```python
from build123d import *

# Parameters (mm, degrees)
BOSS_EXTRUDE1_DEPTH = 2.5
SKETCH2_R           = 1.75
SKETCH2_W           = 3.5
SKETCH2_H           = 6.7
CUT_EXTRUDE1_DEPTH  = 2.5


with BuildPart() as part:
    # Sketch1 → Boss-Extrude1 (new body)
    with BuildSketch(Plane(origin=(0, 0, 0), x_dir=(1, 0, 0), z_dir=(0, 1, 0))):
        Polygon((5.3, 0), (-5.3, 0), (-5.3, 41.8), (-7.6, 41.8), (-7.6, 46.6), (7.6, 46.6), (7.6, 41.8), (5.3, 41.8), align=None)
    extrude(amount=BOSS_EXTRUDE1_DEPTH)

    # Sketch2 → Cut-Extrude1 (cut)
    with BuildSketch(Plane(origin=(0, 0, 0), x_dir=(1, 0, 0), z_dir=(0, 1, 0))):
        with Locations((0, 3.2)):
            Circle(SKETCH2_R)
        with Locations((0, 20.75)):
            Rectangle(SKETCH2_W, SKETCH2_H)
    extrude(amount=CUT_EXTRUDE1_DEPTH, mode=Mode.SUBTRACT)


solid = part.part
```
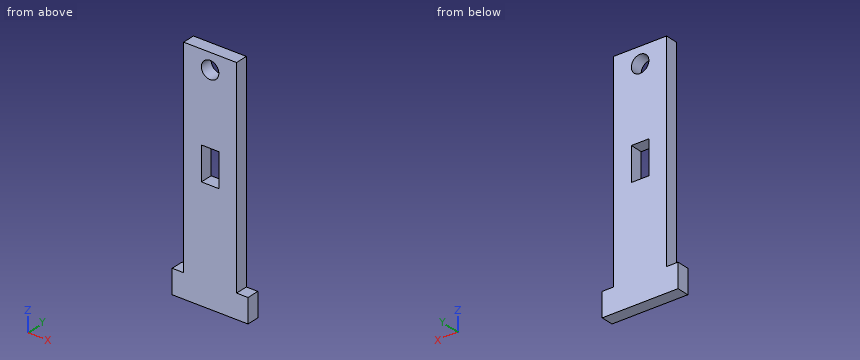
Source: CAD feature listing. Evaluate the final solid. Frame: model axes, mm. Give positions to 0.01 mm unless a question says otherwise; leave off trailing zeros. Loops run counter-clockwise (first coordinate to the right, second up) from the corner with the lowest first, then second, coordinate; pieces in that order, holes last. Notation, with made-up numbers: (39.5, -20) -> (60.5, -20) arc R5 cw to (60.5, -16) -> close; hole circle Ø1 at (-8.75, 34). An arc over 180 degrees is marked (long way). Use a Markdown table: item, result. Add a question column.
(1) Section query D-D (z = -31.5). Output: boundary loops of the cut face in (x, y), then the cut area to 3 significant figures.
(2) Section query A-A (x = 0). Output: boundary loops of the cut face in (y, z), then the cut area to 3 significant figures.
(3) First-contact query: pin 1 Ø1 at (y, z) = (0.5, -10.5) entering from +X; pin 2 Ø0.8 at (y, z) = (1.5, -19) entering from -X; pin 3 Ø1.2 at (x, y) = (-7, 1) entering from +Z; pin 4 Ø3 at (x, z) = (0, -3.2) entering from +Y. Flat tips, straight axial feed; report the tip coordinate or a pass-through.
(4) Ray query, line 1 (Z direction, x = 0, y = 0.75); line 2 (X direction, y = 1.85, z = -3.2). Return the intervals inside material, ascending.
(5) Section query C-C (y = 1.9). Output: boundary loops of the cut face in (x, z).
(6) Section query B-B (z = -3.2). Output: boundary loops of the cut face in (x, y).
Checked values:
| question | item | result |
|---|---|---|
| 1 | outline | (-5.3, 0) -> (5.3, 0) -> (5.3, 2.5) -> (-5.3, 2.5) -> close |
| 1 | area | 26.5 mm^2 |
| 2 | outline | (0, -46.6) -> (2.5, -46.6) -> (2.5, -24.1) -> (0, -24.1) -> close; (0, -17.4) -> (2.5, -17.4) -> (2.5, -4.95) -> (0, -4.95) -> close; (0, -1.45) -> (2.5, -1.45) -> (2.5, 0) -> (0, 0) -> close |
| 2 | area | 91.0 mm^2 |
| 3 | pin 1 | x = 5.3 |
| 3 | pin 2 | x = -5.3 |
| 3 | pin 3 | z = -41.8 |
| 3 | pin 4 | through |
| 4 | line 1 | -46.6 to -24.1, -17.4 to -4.95, -1.45 to 0 |
| 4 | line 2 | -5.3 to -1.75, 1.75 to 5.3 |
| 5 | outline | (-7.6, -46.6) -> (7.6, -46.6) -> (7.6, -41.8) -> (5.3, -41.8) -> (5.3, 0) -> (-5.3, 0) -> (-5.3, -41.8) -> (-7.6, -41.8) -> close; hole (-1.75, -24.1) -> (1.75, -24.1) -> (1.75, -17.4) -> (-1.75, -17.4) -> close; hole circle Ø3.5 at (0, -3.2) |
| 6 | outline | (-5.3, 0) -> (-1.75, 0) -> (-1.75, 2.5) -> (-5.3, 2.5) -> close; (1.75, 0) -> (5.3, 0) -> (5.3, 2.5) -> (1.75, 2.5) -> close |
